from build123d import *

# Parameters (mm, degrees)
F0_W     = 60
F0_H     = 60
F1_DEPTH = 60
F3_D     = 6
F3_DEPTH = 10
F3_TIP   = 1.8025818571
F4_SIZE2 = 50
F4_SIZE  = 20
F5_R     = 14
F6_R     = 9.99999


# Not quite as in the source:
# - a fillet or chamfer is up to 0.001 mm smaller than in the source, because OpenCascade refuses the exact size


with BuildPart() as f1:
    # F0 (on Top) → F1 (new body)
    with BuildSketch(Plane.XY):
        Rectangle(F0_W, F0_H)
    extrude(amount=F1_DEPTH)

    # F3
    with Locations(Plane.XY.offset(60)):
        with Locations((0, 10), (-10, 0), (10, 0), (0, -10), (0, 0)):
            Hole(F3_D / 2, depth=F3_DEPTH)
            with Locations((0, 0, -(F3_DEPTH + F3_TIP / 2))):  # 118° drill point
                Cone(0, F3_D / 2, F3_TIP, mode=Mode.SUBTRACT)

    # F4
    f4_edges = [f1.edges().sort_by_distance(p)[0] for p in [
        (-30, 0, 0),
        (0, -30, 0),
        (30, 0, 0),
        (0, 30, 0),
    ]]
    f4_side = f1.faces().sort_by_distance((0, 0, 0))[0]
    chamfer(f4_edges, length=F4_SIZE, length2=F4_SIZE2, reference=f4_side)

    # F5
    f5_edges = [f1.edges().sort_by_distance(p)[0] for p in [
        (-10, 0, 0),
        (0, 10, 0),
        (0, -10, 0),
        (10, 0, 0),
    ]]
    fillet(f5_edges, radius=F5_R)

    # F6 (radius 10 in the source; OpenCascade refuses exactly that, so slightly less here)
    f6_edges = [f1.edges().sort_by_distance(p)[0] for p in [
        (-30, 0, 60),
        (0, 30, 60),
        (30, 0, 60),
        (0, -30, 60),
    ]]
    fillet(f6_edges, radius=F6_R)


solid = f1.part
The model under review builds one solid part; all positions refer to its coordinate system, in mm. A direction names the side the tool comes from. Round coordinates to 2 decimals unless told otherwise and drop trailing zeros. Write each loop counter-clockwise with the first axis right and the second up, starting at its lowest first coordinate (ties: lowest second). Pieces come first, ordered by that corner, then holes. Notation, with made-up numbers: M 50,-31.75 L 96,-31.75 A26 ccw 96,-1.75 Z; hole C 21,54.25 d5. An arc over 180 degrees is marked long. Use a Markdown table: item, result. Add a question column.
Q1. Insertion check: pin 1 (1.5 mm diameter, centred on x = 17.5, z = 36, fed in from +Y); pin 2 (12 mm diameter, centred on y = 23, z = 10, fed in from +X); pin 3 (2 mm diameter, centred on x = -18.5, y = -23, fed in from +Z); pin 4 (3.5 mm diameter, centred on x = 10, y = 0, fed in from -Z). Each pin has a flat end and moves straight along its axis. Give the tip position at first contact, or say it passes through.
Q2. We need section D-D, the plane z = 40.5. State the section outline as (x, y) points, plus the area to 3 significant figures.
Q3. We need section C-C, the plane z = 32. State the section outline as (x, y) points, plus the area to 3 significant figures.
Q4. The part is to be moulded in two halves that separate along Y. For faces 1 (the face through (3, 0, 55)), 2 (the face through (-27.15, 0.42, 56.99)), 3 (the face through (0.189, 9.743, 3.466)), 4 (the face through (0.24, -10.46, 48.51)), say which applies: pulls with the +Y half, pulls with the -Y half, needs draft (parallel to the pull), parting line crosses it, or undercut.
Q5. To check wall thickness, follow line 1 (X direction, y = 0, z = 57); line 2 (X direction, y = 0, z = 54); line 3 (Y direction, x = 0, z = 55.75). State the ranges of each line that lie inside material, in increasing order.
Q6. Machinability: for faces 5 (the face through (0.189, -9.917, 3.621)), 6 (the face through (12.4, -1.8, 54.9)), which of the approach directions +Z, -Z, +X, -X, +Y, -Y give a long, thin tool a straight path to every point of the face, cutting with its end or side? Answer none if there is none.
Findings below:
| question | item | result |
|---|---|---|
| 1 | pin 1 | stops at y = 24.7 |
| 1 | pin 2 | passes through |
| 1 | pin 3 | stops at z = 59.8 |
| 1 | pin 4 | stops at z = 2.33 |
| 2 | outline | M -26.2,-26.2 L 26.2,-26.2 L 26.2,26.2 L -26.2,26.2 Z |
| 2 | area | 2,750 mm² |
| 3 | outline | M -22.8,-22.8 L 22.8,-22.8 L 22.8,22.8 L -22.8,22.8 Z |
| 3 | area | 2,080 mm² |
| 4 | face 1 | undercut |
| 4 | face 2 | needs draft |
| 4 | face 3 | pulls with the +Y half |
| 4 | face 4 | undercut |
| 5 | line 1 | x = -27.14 to -13, -7 to -3, 3 to 7, 13 to 27.14 |
| 5 | line 2 | x = -29.17 to -13, -7 to -3, 3 to 7, 13 to 29.17 |
| 5 | line 3 | y = -28.18 to -13, -7 to -3, 3 to 7, 13 to 28.18 |
| 6 | face 5 | -Z, +X, -X, -Y |
| 6 | face 6 | +Z |
